Check sheet for the modelled part. Datum: model origin and axes. Units: mm. Face numbers are marked on the shaded views. A direction names the side the tool comes from. Round coordinates to 2 decimals unless told otherwise and drop trailing zeros. Write each loop counter-clockwise with the first axis right and the second up, starting at its lowest first coordinate (ties: lowest second). Pieces come first, ordered by that corner, then holes. Notation, with made-up numbers: M 83,14.25 L 104,14.25 A23 cw 104,42.25 Z; hole C 27.25,44.5 d6. An arc over 180 degrees is marked long. Put each result on its own line as item: value.
```python
from build123d import *

# Parameters (mm, degrees)
SKETCH1_R               = 0.875
BOSS_EXTRUDE1_DEPTH     = 5
CUT_EXTRUDE1_DEPTH      = 6.150849445
CUT_EXTRUDE1_DEPTH_BACK = 6.150849445
SKETCH3_R               = 1.5
BOSS_EXTRUDE2_DEPTH     = 1


with BuildPart() as part:
    # Sketch1 → Boss-Extrude1 (new, symmetric)
    with BuildSketch(Plane(origin=(0, 0, 0), x_dir=(0, 0, -1), z_dir=(1, 0, 0))):
        Circle(SKETCH1_R)
    extrude(amount=BOSS_EXTRUDE1_DEPTH, both=True)

    # Sketch2 → Cut-Extrude1 (cut, two sides: drawn at the far end of the back side and taken through both)
    with BuildSketch(Plane.XY.offset(-CUT_EXTRUDE1_DEPTH_BACK)):
        Polygon((-5, 0.875), (-5, -0.875), (-3.989637029, 0.875), align=None)
        Polygon((5, 0.875), (3.989637029, 0.875), (5, -0.875), align=None)
    extrude(amount=CUT_EXTRUDE1_DEPTH + CUT_EXTRUDE1_DEPTH_BACK, mode=Mode.SUBTRACT)

    # Sketch3 → Boss-Extrude2 (add)
    with BuildSketch(Plane(origin=(3.371113886, 1.946313509, 0), x_dir=(0, 0, -1), z_dir=(0.866025403784438, 0.5000000000000012, 0))):
        with Locations(Location((0, -2.247409257, 0), (0, 0, 90))):
            Circle(SKETCH3_R)
    extrude(amount=BOSS_EXTRUDE2_DEPTH)


solid = part.part
```
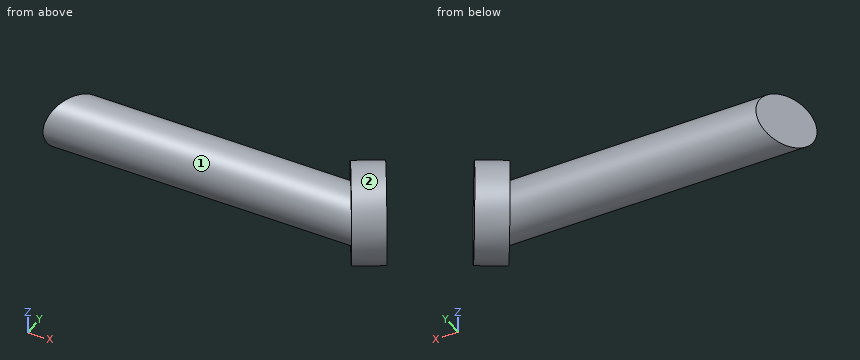
1. Cross-section at B-B (x = -2.5). Enter the section's corners in (y, z) (3 decimals), then the cut area to 3 significant figures.
Computed values:
outline: C 0,0 d1.75
area: 2.41 mm2
2. Scan lines: probe 1 along Z at (x, y) = (3.5, -0.05); probe 2 along Z at (x, y) = (3.25, 0.5); probe 3 along X at (y, z) = (0.1, -0.5). Record each from-to range of solid material in increasing order.
Computed values:
probe 1: z = -0.87 to 0.87
probe 2: z = -0.72 to 0.72
probe 3: x = -4.44 to 5.59
3. Cross-section at D-D (z = 1.25). Enter the section's corners in (x, y).
Computed values:
outline: M 4.08,0.72 L 4.91,-0.72 L 5.78,-0.22 L 4.95,1.22 Z
4. Access from +Z, -Z, +X, -X, +Y, -Y to the whole of each face (thin tool, end or side, straight path). Record for the marked faces 1 and 2.
Computed values:
face 1: -X
face 2: none
5. Cross-section at A-A (z = 0). Enter the section's corners in (x, y) (3 decimals), then the cut area to 3 significant figures.
Computed values:
outline: M -5,-0.875 L 5,-0.875 L 5.245,-1.299 L 6.111,-0.799 L 4.611,1.799 L 3.745,1.299 L 3.99,0.875 L -3.99,0.875 Z
area: 18.7 mm2
6. Cross-section at C-C (z = 0.75). Enter the section's corners in (x, y) (3 decimals).
Computed values:
outline: M -4.755,-0.451 L 4.755,-0.451 L 5.144,-1.125 L 6.01,-0.625 L 4.711,1.625 L 3.845,1.125 L 4.235,0.451 L -4.235,0.451 Z
